Part model, mm, in its own coordinate system. Face numbers are marked on the shaded views. A direction names the side the tool comes from. Coordinates: 2 decimals unless noted, no trailing zeros. Loops run counter-clockwise (first coordinate to the right, second up) from the corner with the lowest first, then second, coordinate; pieces in that order, holes last. Notation, with made-up numbers: M -14.75,43 L 33.25,43 A13 ccw 33.25,52 Z; hole C -15,6.25 d4. An arc over 180 degrees is marked long. Answer as a JSON object with one key per item and string values. Group by question number.
1. Saw through at D-D on x = -54. Write the cut outline in (y, z), then the cut area to 3 significant figures.
2. Saw through at B-B on x = 44. Write the cut outline in (y, z).
3. Mould opens along Z. For the marked faces 3, 4 and 5 say: released by +Z, released by -Z, zero draft, split by the parting line, or undercut.
4. 3-axis set-ups, long thin cutter, end or side, ignore diameter. For the marked faces 1 and 2: which of +Z, -Z, +X, -X, +Y, -Y reach the whole face in a straight line?
5. Saw through at A-A on y = -10. Write the cut outline in (x, z).
6. Drop flat-ended pins along their axis: pin 1 Ø23 at (x, z) = (-11.5, -32) entering from -Y; pin 2 Ø23.5 at (x, z) = (-4, 9.5) entering from -Y. Give the stop position or say it passes through.
7. Saw through at C-C on y = -2.75. Write the cut outline in (x, z).
8. Drill centre lines: L1, parallel to Z at x = 20, y = -7; L2, parallel to X at y = -13.5, z = 27; L3, parallel to X at y = -11.5, z = 71. Where is each one in solid material? Low to high.
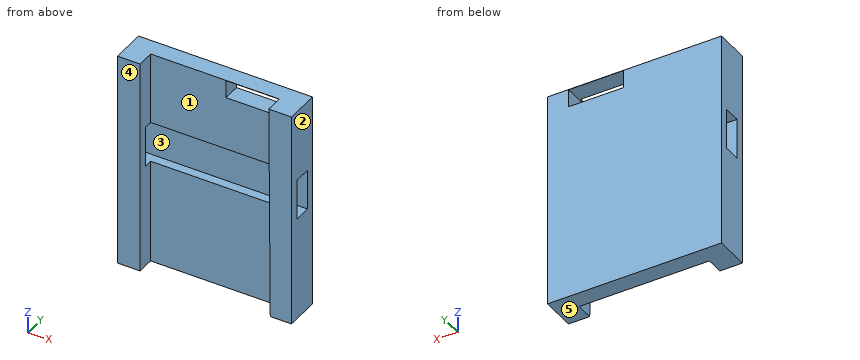
from build123d import *

# Parameters (mm, degrees)
F0_W     = 127
F0_H     = 158.242
F1_DEPTH = 25.4
F4_DEPTH = 12.7
F5_W     = 40
F5_H     = 13
F6_DEPTH = 25
F7_W     = 12.711242
F7_H     = 29.659567
F8_DEPTH = 152.4


with BuildPart() as f1:
    # F0 (on Front) → F1 (new body)
    with BuildSketch(Plane.XZ):
        Rectangle(F0_W, F0_H)
    extrude(amount=F1_DEPTH)

    # F3 (on face) → F4 (cut)
    with BuildSketch(Plane.XZ.offset(25.4)):
        Polygon((48.082705, -86.58883), (46.892088, 91.21117), (-46.977836, 91.21117), (-46.977836, -86.58883), align=None)
    extrude(amount=-F4_DEPTH, mode=Mode.SUBTRACT)

    # F5 (on face) → F6 (cut)
    with BuildSketch(Plane(origin=(0, 0, 0), x_dir=(-1, 0, 0), z_dir=(0, 1, 0))):
        with Locations((-28.005632, 72.421707)):
            Rectangle(F5_W, F5_H)
    extrude(amount=-F6_DEPTH, mode=Mode.SUBTRACT)

    # F7 (on face) → F8 (cut)
    with BuildSketch(Plane.YZ.offset(63.5)):
        with Locations((-12.408594, 11.954622)):
            Rectangle(F7_W, F7_H)
    extrude(amount=-F8_DEPTH, mode=Mode.SUBTRACT)


solid = f1.part
Outcome:
{
 "1": {"outline": "M -25.4,-79.12 L 0,-79.12 L 0,79.12 L -25.4,79.12 Z; hole M -18.76,-2.88 L -6.05,-2.88 L -6.05,26.78 L -18.76,26.78 Z", "area": "3,640 mm²"},
 "2": {"outline": "M -12.7,-79.12 L 0,-79.12 L 0,65.92 L -12.7,65.92 L -12.7,26.78 L -6.05,26.78 L -6.05,-2.88 L -12.7,-2.88 Z; M -12.7,78.92 L 0,78.92 L 0,79.12 L -12.7,79.12 Z"},
 "3": {"face 3": "undercut", "face 4": "zero draft", "face 5": "released by -Z"},
 "4": {"face 1": "+Z, -Z, -Y", "face 2": "+Z, -Z, +X, +Y, -Y"},
 "5": {"outline": "M -63.5,-79.12 L 63.5,-79.12 L 63.5,-2.88 L -63.5,-2.88 Z; M -63.5,26.78 L 63.5,26.78 L 63.5,79.12 L -63.5,79.12 Z; hole M 8.01,65.92 L 48.01,65.92 L 48.01,78.92 L 8.01,78.92 Z"},
 "6": {"pin 1": "stops at y = -12.7", "pin 2": "stops at y = -6.05"},
 "7": {"outline": "M -63.5,-79.12 L 63.5,-79.12 L 63.5,79.12 L -63.5,79.12 Z; hole M 8.01,65.92 L 48.01,65.92 L 48.01,78.92 L 8.01,78.92 Z"},
 "8": {"L1": "z = -79.12 to -2.88, 26.78 to 65.92, 78.92 to 79.12", "L2": "x = -63.5 to -46.98, 47.32 to 63.5", "L3": "x = -63.5 to 8.01, 48.01 to 63.5"}
}
